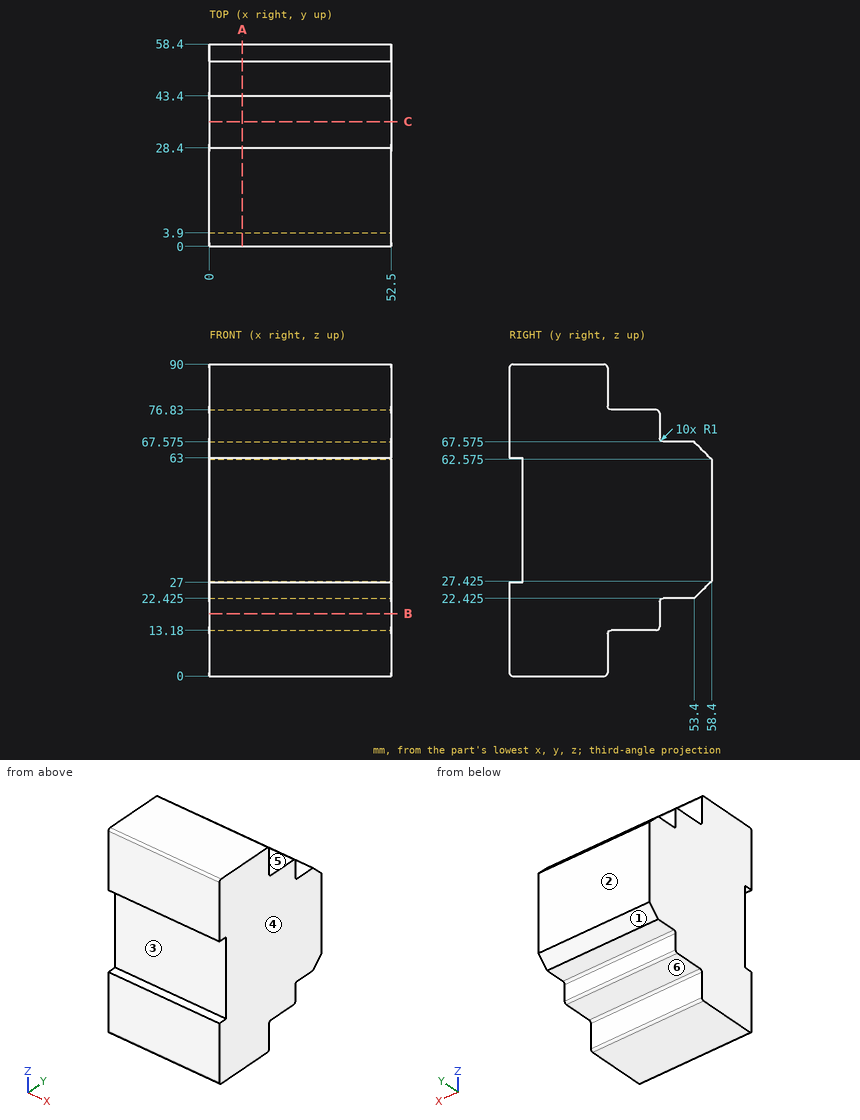
Design review of the part shown in the three views and the two pictorial views. Dimensions are in mm from the part's minimum x, y and z. A direction names the side the tool comes from. Coordinates: 2 decimals unless noted, no trailing zeros. Order: outer loops, then holes, each group sorted by start corner. A loop starts at its lowest first (then second) coordinate and runs counter-clockwise, first axis right, second up.
1) For the marked faces 4, 5 and 6, list the 3-axis set-ups (+Z, -Z, +X, -X, +Y, -Y) from which the entire face can be reached by the end or side of a thin tool; tool diameter is ignored.
2) Mouldability with a two-part tool opening along Z and no side actions: class the marked faces 1, 2 and 3 as +Z half, -Z half, draft (parallel to the pull), parting line (faces both ways), or undercut.
3) Clearance check with flat-ended pins moving along their axes: pin 1 (9 mm diameter, centred on x = 14.5, z = 86, fed in from +Y); pin 2 (6 mm diameter, centred on x = 13.5, y = 32, fed in from +Z); pin 3 (11 mm diameter, centred on x = 28, z = 50, fed in from -Y); pin 4 (14.5 mm diameter, centred on x = 17, y = 34.5, fed in from -Z). State where each tip first meets the part, or that it passes through.
4) Take a section at A-A, the plane x = 9.5. Give the boundary of the cut face in (y, z) (3 decimals).
5) Take a section at B-B, the plane z = 18. Give the boundary of the cut face in (x, y), and give its area (3 significant figures).
6) Wall thickness on line 1 along Y through (x, z) = (11, 39); line 2 along Z through (x, y) = (6, 32.5); line 3 along Y through (x, z) = (40, 17): over which ranges is each line inside the solid? List them lowest first.
7) Take a section at C-C, the plane y = 36. Give the boundary of the cut face in (x, z), and give its area (3 significant figures).
Returned:
1. face 4: +Z, -Z, +X, +Y, -Y
1. face 5: +Z, +X, -X, +Y
1. face 6: -Z, +X, -X, +Y
2. face 1: -Z half
2. face 2: draft
2. face 3: undercut
3. pin 1: stops at y = 28.4
3. pin 2: stops at z = 76.91
3. pin 3: stops at y = 3.9
3. pin 4: stops at z = 0
4. outline: (0, 1) arc R1 ccw to (1, 0) - (27.4, 0) arc R1 ccw to (28.4, 1) - (28.4, 12.18) arc R1 cw to (29.4, 13.18) - (42.4, 13.18) arc R1 ccw to (43.4, 14.18) - (43.4, 21.425) arc R1 cw to (44.4, 22.425) - (53.4, 22.425) - (58.4, 27.425) - (58.4, 62.575) - (53.4, 67.575) - (44.4, 67.575) arc R1 cw to (43.4, 68.575) - (43.4, 75.83) arc R1 ccw to (42.4, 76.83) - (29.4, 76.83) arc R1 cw to (28.4, 77.83) - (28.4, 89) arc R1 ccw to (27.4, 90) - (1, 90) arc R1 ccw to (0, 89) - (0, 63) - (3.9, 63) - (3.9, 27) - (0, 27) - close
5. outline: (0, 0) - (52.5, 0) - (52.5, 43.4) - (0, 43.4) - close
5. area: 2,280 mm2
6. line 1: y = 3.9 to 58.4
6. line 2: z = 13.18 to 76.83
6. line 3: y = 0 to 43.4
7. outline: (0, 13.18) - (52.5, 13.18) - (52.5, 76.83) - (0, 76.83) - close
7. area: 3,340 mm2
